from build123d import *

# Parameters (mm, degrees)
P_IDAT_VYSUNUT_M1_DEPTH                           = 4
KU_ELOV_ZAHLOUBEN_PRO_M3_ROUBU_SE_Z_P_D           = 3.4
KU_ELOV_ZAHLOUBEN_PRO_M3_ROUBU_SE_Z_P_CSINK_D     = 6.3
KU_ELOV_ZAHLOUBEN_PRO_M3_ROUBU_SE_Z_P_CSINK_ANGLE = 90
ZKOSEN_1_SIZE                                     = 1
SKICA4_W                                          = 6.6
SKICA4_H                                          = 14.2
ODEBRAT_VYSUNUT_M1_DEPTH                          = 91.589306764


with BuildPart() as part:
    # Skica1 → Přidat vysunutím1 (new body)
    with BuildSketch(Plane(origin=(0, 0, -86), x_dir=(-1, 0, 0), z_dir=(0, 0, -1))):
        with BuildLine():
            Line((-75, 44.35), (-75, -45.65))
            ThreePointArc((-75, -45.65), (-73.535533906, -49.185533906), (-70, -50.65))
            Line((-70, -50.65), (70, -50.65))
            ThreePointArc((70, -50.65), (73.535533906, -49.185533906), (75, -45.65))
            Line((75, -45.65), (75, 44.35))
            ThreePointArc((75, 44.35), (73.535533906, 47.885533906), (70, 49.35))
            Line((70, 49.35), (-70, 49.35))
            ThreePointArc((-70, 49.35), (-73.535533906, 47.885533906), (-75, 44.35))
        make_face()
    extrude(amount=P_IDAT_VYSUNUT_M1_DEPTH)

    # Kuželové zahloubení pro M3 šroubu se zápustnou hlavou plochou1 (through all)
    with Locations(Plane(origin=(0, 0, -90), x_dir=(-1, 0, 0), z_dir=(0, 0, -1))):
        with Locations((70, -45.657811951), (70, 44.357811951), (-70, 44.357811951), (-70, -45.657811951)):
            CounterSinkHole(KU_ELOV_ZAHLOUBEN_PRO_M3_ROUBU_SE_Z_P_D / 2, KU_ELOV_ZAHLOUBEN_PRO_M3_ROUBU_SE_Z_P_CSINK_D / 2, counter_sink_angle=KU_ELOV_ZAHLOUBEN_PRO_M3_ROUBU_SE_Z_P_CSINK_ANGLE)

    # Zkosení1
    zkosen_1_edges = [part.edges().sort_by_distance(p)[0] for p in [
        (73.535533906, -49.185533906, -90),
        (0, -50.65, -90),
        (-73.535533906, -49.185533906, -90),
        (-75, -0.65, -90),
        (-73.535533906, 47.885533906, -90),
        (0, 49.35, -90),
        (73.535533906, 47.885533906, -90),
        (75, -0.65, -90),
    ]]
    chamfer(zkosen_1_edges, length=ZKOSEN_1_SIZE)

    # Skica4 → Odebrat vysunutím1 (cut, through all)
    with BuildSketch(Plane(origin=(0, 0, -90), x_dir=(-1, 0, 0), z_dir=(0, 0, -1))):
        with Locations((65.2, -29.5)):
            Rectangle(SKICA4_W, SKICA4_H)
        with Locations((65.2, -9.4)):
            Rectangle(SKICA4_W, SKICA4_H)
        with Locations((65.2, 10.6)):
            Rectangle(SKICA4_W, SKICA4_H)
    extrude(amount=-ODEBRAT_VYSUNUT_M1_DEPTH, mode=Mode.SUBTRACT)


solid = part.part
The model under review builds one solid part; all positions refer to its coordinate system, in mm. A direction names the side the tool comes from. Round coordinates to 2 decimals unless told otherwise and drop trailing zeros. Write each loop counter-clockwise with the first axis right and the second up, starting at its lowest first coordinate (ties: lowest second). Pieces come first, ordered by that corner, then holes. Notation, with made-up numbers: M -19.5,84 L 22.5,84 A25 ccw 22.5,103 Z; hole C 3,77.5 d1. An arc over 180 degrees is marked long. Use a Markdown table: item, result. Add a question column.
Q1. We need section B-B, the plane z = -87. State the section outline as (x, y) points.
Q2. Insertion check: pin 1 (5.5 mm diameter, centred on x = -70, y = 44.36, fed in from -Z); pin 2 (2 mm diameter, centred on x = 70, y = 44.36, fed in from -Z). Each pin has a flat end and moves straight along its axis. Give the tip position at first contact, or say it passes through.
Q3. To check wall thickness, follow line 1 (Y direction, x = -70, z = -87.35); line 2 (X direction, y = -13.5, z = -88.05); line 3 (Y direction, x = 68.5, z = -89.3). State the ranges of each line that lie inside material, in increasing order.
Q4. We need section A-A, the plane y = 5.5. State the section outline as (x, z) points.
Q5. Machinability: for faces 5 (the face through (73.57, -49.15, -87.48)), 6 (the face through (-61.9, -30, -88)), which of the approach directions +Z, -Z, +X, -X, +Y, -Y give a long, thin tool a straight path to every point of the face, cutting with its end or side? Answer none if there is none.
Q6. The part is to be moulded in two halves that separate along X. For faces 1 (the face through (75, 0, -87)), 2 (the face through (1, 0, -90)), 3 (the face through (68.651, 43.323, -87.257)), 4 (the face through (-75, -1, -87)), say which applies: pulls with the +X half, pulls with the -X half, needs draft (parallel to the pull), parting line crosses it, or undercut.
Findings below:
| question | item | result |
|---|---|---|
| 1 | outline | M -75,-45.65 A5 ccw -70,-50.65 L 70,-50.65 A5 ccw 75,-45.65 L 75,44.35 A5 ccw 70,49.35 L -70,49.35 A5 ccw -75,44.35 Z; hole C -70,-45.66 d3.4; hole C -70,44.36 d3.4; hole M -68.5,-36.6 L -61.9,-36.6 L -61.9,-22.4 L -68.5,-22.4 Z; hole M -68.5,-16.5 L -61.9,-16.5 L -61.9,-2.3 L -68.5,-2.3 Z; hole M -68.5,3.5 L -61.9,3.5 L -61.9,17.7 L -68.5,17.7 Z; hole C 70,-45.66 d3.4; hole C 70,44.36 d3.4 |
| 2 | pin 1 | stops at z = -89.6 |
| 2 | pin 2 | passes through |
| 3 | line 1 | y = -50.65 to -47.36, -43.96 to 42.66, 46.06 to 49.35 |
| 3 | line 2 | x = -75 to -68.5, -61.9 to 75 |
| 3 | line 3 | y = -50.35 to -47.59, -43.72 to 42.42, 46.29 to 49.05 |
| 4 | outline | M -75,-89 L -74,-90 L -68.5,-90 L -68.5,-86 L -75,-86 Z; M -61.9,-90 L 74,-90 L 75,-89 L 75,-86 L -61.9,-86 Z |
| 5 | face 5 | +Z, -Z, +X, -Y |
| 5 | face 6 | +Z, -Z |
| 6 | face 1 | pulls with the +X half |
| 6 | face 2 | needs draft |
| 6 | face 3 | undercut |
| 6 | face 4 | pulls with the -X half |
